from build123d import *

# Parameters (mm, degrees)
SKETCH1_R           = 20.41525
SKETCH1_R_2         = 16.79575
BOSS_EXTRUDE1_DEPTH = 28.8925
SKETCH2_R           = 20.41525
SKETCH2_R_2         = 16.09725
REVOLVE1_ANGLE      = 90
SKETCH3_R           = 20.41525
SKETCH3_R_2         = 16.79575
BOSS_EXTRUDE2_DEPTH = 28.8925
SKETCH5_W           = 42.418
SKETCH5_H           = 19.05
CUT_EXTRUDE2_DEPTH  = 66.9925


with BuildPart() as part:
    # Sketch1 → Boss-Extrude1 (new body)
    with BuildSketch(Plane(origin=(0, 0, 0), x_dir=(1, 0, 0), z_dir=(0, 1, 0))):
        Circle(SKETCH1_R)
        Circle(SKETCH1_R_2, mode=Mode.SUBTRACT)
    extrude(amount=BOSS_EXTRUDE1_DEPTH)

    # Sketch2 → Revolve1 (revolve)
    with BuildSketch(Plane(origin=(0, 28.8925, 0), x_dir=(1, 0, 0), z_dir=(0, 1, 0))):
        Circle(SKETCH2_R)
        Circle(SKETCH2_R_2, mode=Mode.SUBTRACT)
    revolve(axis=Axis((23.59025, 28.8925, 20.41525), (0, 0, -1)), revolution_arc=REVOLVE1_ANGLE)

    # Sketch3 → Boss-Extrude2 (add)
    with BuildSketch(Plane(origin=(23.59025, 0, 0), x_dir=(0, 0, -1), z_dir=(1, 0, 0))):
        with Locations((0, 52.48275)):
            Circle(SKETCH3_R)
        with Locations((0, 52.48275)):
            Circle(SKETCH3_R_2, mode=Mode.SUBTRACT)
    extrude(amount=BOSS_EXTRUDE2_DEPTH)

    # Sketch5 → Cut-Extrude2 (cut)
    with BuildSketch(Plane(origin=(0, 28.8925, -20.41525), x_dir=(-1, 0, 0), z_dir=(0, 0, -1))):
        with Locations((-0.79375, 34.4805)):
            Rectangle(SKETCH5_W, SKETCH5_H)
    extrude(amount=-CUT_EXTRUDE2_DEPTH, mode=Mode.SUBTRACT)


solid = part.part
Read the model definition and answer for the solid it produces. Units are mm, in the model's axes. A direction names the side the tool comes from. Round coordinates to 2 decimals unless told otherwise and drop trailing zeros. Loops run counter-clockwise (first coordinate to the right, second up) from the corner with the lowest first, then second, coordinate; pieces in that order, holes last.
Q1. Each of these flat-tipped pins is pushed along its axis until it touches: pin 1 (8 mm diameter, centred on x = 26, y = 63.5, fed in from +Z); pin 2 (10 mm diameter, centred on x = -3, z = 7.5, fed in from +Y); pin 3 (3 mm diameter, centred on x = -3, z = 6, fed in from +Y); pin 4 (10 mm diameter, centred on y = 45, z = 2, fed in from +X). Where does it stop, or does it pass through?
Q2. Which of the six approach directions +Z, -Z, +X, -X, +Y, -Y give full straight-line access (tool end or side, diameter ignored) to faces 5 (the face through (37.834, 69.136, 2.186)), 6 (the face through (3, 0, 17)), 7 (the face through (22.003, 69, -2))?
Q3. Determine the mould class of faces 1 (the face through (23.59, 44, 14)), 2 (the face through (-2.66, 14.24, -20.24)), 3 (the face through (9, 28.892, 14)), 4 (the face through (-3.641, 14.244, 16.396)) for opening direction X: released by +X, released by -X, zero draft, split by the parting line, or undercut.
Q4. Section A-A on z = -8.5 is taken. Write down the section's boundary in (x, y).
Q5. Consider probe 1 along Y at (x, z) = (36, 0); probe 2 along Z at (x, y) = (0, 8). Determine where each line is inside the solid, lowest interval first.
Q6. Section C-C on z = 3 is taken. Write down the section's boundary in (x, y), and give its area (3 significant figures).
Q7. Section B-B on y = 27.5 is taken. Write down the section's boundary in (x, z), and give its area (3 significant figures).
Output:
1. pin 1: stops at z = 19.17
1. pin 2: stops at y = 53.85
1. pin 3: passes through
1. pin 4: stops at x = -9.68
2. face 5: +X
2. face 6: +Z, -Z, +X, -X, -Y
2. face 7: +Z, -Z, -X, +Y
3. face 1: released by +X
3. face 2: split by the parting line
3. face 3: undercut
3. face 4: undercut
4. outline: (-18.56, 0) - (-14.49, 0) - (-14.49, 28.89) - (-13.67, 28.89) arc R37.26 cw to (-4.08, 53.85) - (-10.38, 53.85) arc R42.15 ccw to (-18.56, 28.89) - close; (13.67, 28.89) - (14.49, 28.89) - (14.49, 0) - (18.56, 0) - (18.56, 28.89) arc R5.03 cw to (23.59, 33.92) - (52.48, 33.92) - (52.48, 38) - (23.59, 38) - (23.59, 38.81) arc R9.92 ccw to start; (22, 66.12) arc R37.26 cw to (23.59, 66.15) - (23.59, 66.97) - (52.48, 66.97) - (52.48, 71.04) - (23.59, 71.04) arc R42.15 ccw to (22, 71.01) - close
5. probe 1: y = 32.07 to 35.69, 69.28 to 72.9
5. probe 2: z = -20.42 to -16.8, 16.8 to 20.42
6. outline: (-20.19, 0) - (-16.53, 0) - (-16.53, 28.89) - (-15.82, 28.89) arc R39.41 cw to (-6.91, 53.85) - (-12.39, 53.85) arc R43.78 ccw to (-20.19, 28.89) - close; (15.82, 28.89) - (16.53, 28.89) - (16.53, 0) - (20.19, 0) - (20.19, 28.89) arc R3.4 cw to (23.59, 32.29) - (52.48, 32.29) - (52.48, 35.96) - (23.59, 35.96) - (23.59, 36.67) arc R7.78 ccw to start; (22, 68.27) arc R39.41 cw to (23.59, 68.3) - (23.59, 69.01) - (52.48, 69.01) - (52.48, 72.68) - (23.59, 72.68) arc R43.78 ccw to (22, 72.65) - close
6. area: 586 mm2
7. outline: circle Ø40.83 at (0, 0); hole circle Ø33.59 at (0, 0)
7. area: 423 mm2
